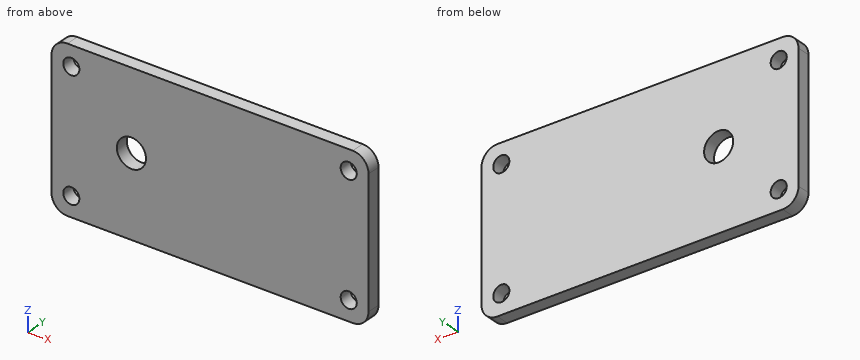
```python
from build123d import *

# Parameters (mm, degrees)
SKETCH1_W               = 120
SKETCH1_H               = 60
BOSS_EXTRUDE1_DEPTH     = 5
SKETCH2_R               = 3.05
CUT_EXTRUDE1_DEPTH      = 68.268120235
MIRROR2_COPY_1_SKETCH_R = 3.05
MIRROR2_COPY_1_DEPTH    = 68.268120235
SKETCH3_R               = 5.5
CUT_EXTRUDE2_DEPTH      = 68.268120235
FILLET1_R               = 6


with BuildPart() as part:
    # Sketch1 → Boss-Extrude1 (new body)
    with BuildSketch(Plane(origin=(0, 0, 0), x_dir=(1, 0, 0), z_dir=(0, 1, 0))):
        Rectangle(SKETCH1_W, SKETCH1_H)
    extrude(amount=BOSS_EXTRUDE1_DEPTH)

    # Sketch2 → Cut-Extrude1 (cut, through all)
    with BuildSketch(Plane(origin=(0, 5, 0), x_dir=(1, 0, 0), z_dir=(0, 1, 0))):
        with Locations(Location((-52.5, 22.5, 0), (0, 0, 270))):
            Circle(SKETCH2_R)
    cut_extrude1 = extrude(amount=-CUT_EXTRUDE1_DEPTH, mode=Mode.SUBTRACT)

    # Mirror1: Cut-Extrude1 across plane
    add(cut_extrude1.mirror(Plane.XY), mode=Mode.SUBTRACT)

    # Mirror2: Cut-Extrude1 across plane
    add(cut_extrude1.mirror(Plane(origin=(0, 0, 0), x_dir=(0, 0, 1), z_dir=(1, 0, 0))), mode=Mode.SUBTRACT)

    # Mirror2 copy 1 sketch → Mirror2 copy 1 (cut, through all)
    with BuildSketch(Plane(origin=(0, 5, 0), x_dir=(-1, 0, 0), z_dir=(0, 1, 0))):
        with Locations(Location((-52.5, 22.5, 0), (0, 0, 270))):
            Circle(MIRROR2_COPY_1_SKETCH_R)
    extrude(amount=-MIRROR2_COPY_1_DEPTH, mode=Mode.SUBTRACT)

    # Sketch3 → Cut-Extrude2 (cut, through all)
    with BuildSketch(Plane(origin=(0, 5, 0), x_dir=(1, 0, 0), z_dir=(0, 1, 0))):
        with Locations(Location((-29.74982269, -0.203269064, 0), (0, 0, 270))):
            Circle(SKETCH3_R)
    extrude(amount=-CUT_EXTRUDE2_DEPTH, mode=Mode.SUBTRACT)

    # Fillet1
    fillet1_edges = [part.edges().sort_by_distance(p)[0] for p in [
        (60, 2.5, 30),
        (-60, 2.5, 30),
        (-60, 2.5, -30),
        (60, 2.5, -30),
    ]]
    fillet(fillet1_edges, radius=FILLET1_R)


solid = part.part
```
Can you work these out from the model? Positions are in its coordinate system, mm. Give positions to 0.01 mm unless a question says otherwise; leave off trailing zeros. Order: outer loops, then holes, each group sorted by start corner. A loop starts at its lowest first (then second) coordinate and runs counter-clockwise, first axis right, second up. Notation, with made-up numbers: M 11,80.25 L 37,80.25 A34 ccw 37,118.25 Z; hole C 64,-12.75 d6. An arc over 180 degrees is marked long. Write item = value, one per line. Start each with the question number.
Q1. Suppose I cut it at A-A (z = 22.5). Write out the boundary of the cut face in (x, y).
Q2. Suppose I cut it at C-C (y = 2.35). Write out the boundary of the cut face in (x, z), plus the area to 3 significant figures.
Q3. Suppose I cut it at B-B (x = 52.5). Write out the boundary of the cut face in (y, z).
Q4. I need wall thicknesses on probe 1 along X at (y, z) = (3.95, 22.5); probe 2 along Z at (x, y) = (52.5, 3.9); probe 3 along X at (y, z) = (3.1, 26). Which ranges of each line are inside material? Lowest first, please. Write a range as [from, to].
Check result:
q1.outline = M -60,0 L -55.55,0 L -55.55,5 L -60,5 Z; M -49.45,0 L 49.45,0 L 49.45,5 L -49.45,5 Z; M 55.55,0 L 60,0 L 60,5 L 55.55,5 Z
q2.outline = M -60,-24 A6 ccw -54,-30 L 54,-30 A6 ccw 60,-24 L 60,24 A6 ccw 54,30 L -54,30 A6 ccw -60,24 Z; hole C -52.5,-22.5 d6.1; hole C -52.5,22.5 d6.1; hole C -29.75,0.2 d11; hole C 52.5,-22.5 d6.1; hole C 52.5,22.5 d6.1
q2.area = 6,960 mm2
q3.outline = M 0,-30 L 5,-30 L 5,-25.55 L 0,-25.55 Z; M 0,-19.45 L 5,-19.45 L 5,19.45 L 0,19.45 Z; M 0,25.55 L 5,25.55 L 5,30 L 0,30 Z
q4.probe_1 = [-60, -55.55], [-49.45, 49.45], [55.55, 60]
q4.probe_2 = [-30, -25.55], [-19.45, 19.45], [25.55, 30]
q4.probe_3 = [-59.66, 59.66]
